from build123d import *

# Parameters (mm, degrees)
SKETCH2_R           = 4
SKETCH2_R_2         = 30
SKETCH2_R_3         = 8.623329564
SKETCH2_R_4         = 8.505813098
SKETCH2_R_5         = 8.401963559
SKETCH2_W           = 13
SKETCH2_H           = 48.5
BOSS_EXTRUDE1_DEPTH = 6.35


with BuildPart() as part:
    # Sketch2 → Boss-Extrude1 (new body)
    with BuildSketch(Plane.XY):
        with BuildLine():
            ThreePointArc((80.527805435, 108.72490148), (73, 126.439708953), (53.894623988, 124.101575958))
            ThreePointArc((53.894623988, 124.101575958), (29.058945383, 107.994153026), (0, 102.351662573))
            ThreePointArc((0, 102.351662573), (-29.058945383, 107.994153026), (-53.894623988, 124.101575958))
            ThreePointArc((-53.894623988, 124.101575958), (-73, 126.439708953), (-80.527805435, 108.72490148))
            ThreePointArc((-80.527805435, 108.72490148), (-78.996207289, 79.162861422), (-88.639139908, 51.175831286))
            ThreePointArc((-88.639139908, 51.175831286), (-108.055152672, 28.831291604), (-134.422429423, 15.376674478))
            ThreePointArc((-134.422429423, 15.376674478), (-146, 0), (-134.422429423, -15.376674478))
            ThreePointArc((-134.422429423, -15.376674478), (-108.055152672, -28.831291604), (-88.639139908, -51.175831286))
            ThreePointArc((-88.639139908, -51.175831286), (-78.996207289, -79.162861422), (-80.527805435, -108.72490148))
            ThreePointArc((-80.527805435, -108.72490148), (-73, -126.439708953), (-53.894623988, -124.101575958))
            ThreePointArc((-53.894623988, -124.101575958), (-29.058945383, -107.994153026), (0, -102.351662573))
            ThreePointArc((0, -102.351662573), (29.058945383, -107.994153026), (53.894623988, -124.101575958))
            ThreePointArc((53.894623988, -124.101575958), (73, -126.439708953), (80.527805435, -108.72490148))
            ThreePointArc((80.527805435, -108.72490148), (78.996207289, -79.162861422), (88.639139908, -51.175831286))
            ThreePointArc((88.639139908, -51.175831286), (108.055152672, -28.831291604), (134.422429423, -15.376674478))
            ThreePointArc((134.422429423, -15.376674478), (146, 0), (134.422429423, 15.376674478))
            ThreePointArc((134.422429423, 15.376674478), (108.055152672, 28.831291604), (88.639139908, 51.175831286))
            ThreePointArc((88.639139908, 51.175831286), (78.996207289, 79.162861422), (80.527805435, 108.72490148))
        make_face()
        with Locations((65, 112.583302492)):
            Circle(SKETCH2_R, mode=Mode.SUBTRACT)
        with Locations((130, 0)):
            Circle(SKETCH2_R, mode=Mode.SUBTRACT)
        with Locations((65, -112.583302492)):
            Circle(SKETCH2_R, mode=Mode.SUBTRACT)
        with Locations((-65, -112.583302492)):
            Circle(SKETCH2_R, mode=Mode.SUBTRACT)
        with Locations((-130, 0)):
            Circle(SKETCH2_R, mode=Mode.SUBTRACT)
        with Locations((-65, 112.583302492)):
            Circle(SKETCH2_R, mode=Mode.SUBTRACT)
        with Locations((25.068716778, 29.875733282)):
            Circle(SKETCH2_R, mode=Mode.SUBTRACT)
        with Locations((38.407502367, 6.772278929)):
            Circle(SKETCH2_R, mode=Mode.SUBTRACT)
        with Locations((33.774990748, -19.5)):
            Circle(SKETCH2_R, mode=Mode.SUBTRACT)
        with Locations((13.33878559, -36.648012211)):
            Circle(SKETCH2_R, mode=Mode.SUBTRACT)
        with Locations((-13.33878559, -36.648012211)):
            Circle(SKETCH2_R, mode=Mode.SUBTRACT)
        with Locations((-33.774990748, -19.5)):
            Circle(SKETCH2_R, mode=Mode.SUBTRACT)
        with Locations((-38.407502367, 6.772278929)):
            Circle(SKETCH2_R, mode=Mode.SUBTRACT)
        with Locations((-25.068716778, 29.875733282)):
            Circle(SKETCH2_R, mode=Mode.SUBTRACT)
        Circle(SKETCH2_R_2, mode=Mode.SUBTRACT)
        with Locations((43.278364114, -31.443572071)):
            Circle(SKETCH2_R_3, mode=Mode.SUBTRACT)
        with Locations((53.495, 0)):
            Circle(SKETCH2_R_4, mode=Mode.SUBTRACT)
        with Locations((43.278364114, 31.443572071)):
            Circle(SKETCH2_R_5, mode=Mode.SUBTRACT)
        with Locations((0, 39)):
            Circle(SKETCH2_R, mode=Mode.SUBTRACT)
        with Locations((-13.33878559, 54.898012211)):
            Rectangle(SKETCH2_W, SKETCH2_H, mode=Mode.SUBTRACT)
        with Locations((13.33878559, 54.898012211)):
            Rectangle(SKETCH2_W, SKETCH2_H, mode=Mode.SUBTRACT)
    extrude(amount=BOSS_EXTRUDE1_DEPTH)


solid = part.part
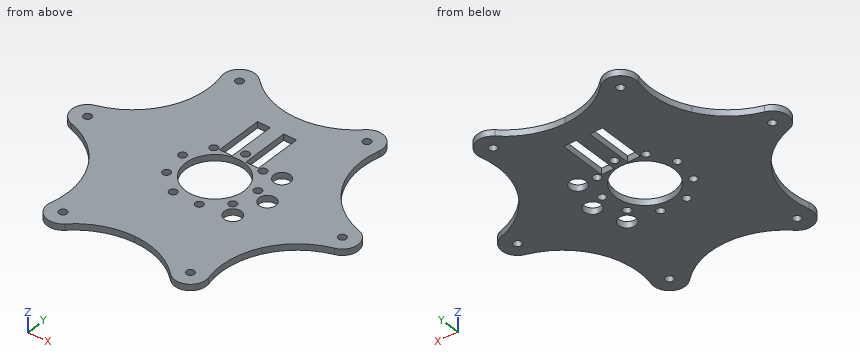
Work out the finished part from the listing and answer in its coordinate system (mm). Give positions to 0.01 mm unless a question says otherwise; leave off trailing zeros. Loops run counter-clockwise (first coordinate to the right, second up) from the corner with the lowest first, then second, coordinate; pieces in that order, holes last. Notation, with made-up numbers: (-18.75, 27) -> (21.25, 27) arc R18 ccw to (21.25, 39) -> close; hole circle Ø6 at (17.25, 57). An arc over 180 degrees is marked (long way). Use a Markdown table: item, result. Add a question column.
1. Flat-ended cylindrical pins translate along their axes: pin 1 Ø1.9 at (x, z) = (-12.5, 3.5) entering from -Y; pin 2 Ø19.5 at (x, y) = (43.28, 31.44) entering from +Z; pin 3 Ø3 at (y, z) = (-13, 1.5) entering from +X; pin 4 Ø1 at (x, z) = (-60, 1) entering from -Y. Find the tip coordinate at first contact, or state that the pin passes through.
2. Find the intervals of material crossed by probe 1 along Y at (x, z) = (-65, 2.5); probe 2 along X at (y, z) = (59.5, 1.25); probe 3 along X at (y, z) = (40.5, 3.5), in increasing order.
3. Section B-B on x = -130 is taken. Determine the outline of the cut face in (y, z).
4. Section C-C on y = -78 is taken. Determine the outline of the cut face in (x, z), and give its area (3 significant figures).
5. Section A-A on x = -65 is taken. Determine the outline of the cut face in (y, z).
6. Section D-D on z = 4 is taken. State how many separate pieces and enclosed holes the cut face has, and give its area (3 significant figures).
Results below:
| question | item | result |
|---|---|---|
| 1 | pin 1 | stops at y = -103.53 |
| 1 | pin 2 | stops at z = 6.35 |
| 1 | pin 3 | stops at x = 141.12 |
| 1 | pin 4 | stops at y = -127.94 |
| 2 | probe 1 | y = -128.58 to -116.58, -108.58 to 108.58, 116.58 to 128.58 |
| 2 | probe 2 | x = -84.48 to -19.84, -6.84 to 6.84, 19.84 to 84.48 |
| 2 | probe 3 | x = -96.06 to -19.84, -6.84 to -3.71, 3.71 to 6.84, 19.84 to 96.06 |
| 3 | outline | (-16.79, 0) -> (-4, 0) -> (-4, 6.35) -> (-16.79, 6.35) -> close; (4, 0) -> (16.79, 0) -> (16.79, 6.35) -> (4, 6.35) -> close |
| 4 | outline | (-79.17, 0) -> (79.17, 0) -> (79.17, 6.35) -> (-79.17, 6.35) -> close |
| 4 | area | 1,010 mm^2 |
| 5 | outline | (-128.58, 0) -> (-116.58, 0) -> (-116.58, 6.35) -> (-128.58, 6.35) -> close; (-108.58, 0) -> (108.58, 0) -> (108.58, 6.35) -> (-108.58, 6.35) -> close; (116.58, 0) -> (128.58, 0) -> (128.58, 6.35) -> (116.58, 6.35) -> close |
| 6 | separate pieces | 1 |
| 6 | enclosed holes | 21 |
| 6 | area | 38,900 mm^2 |
